Verification items for the finished model (mm, model axes). A direction names the side the tool comes from. Coordinates: 2 decimals unless noted, no trailing zeros. Write each loop counter-clockwise with the first axis right and the second up, starting at its lowest first coordinate (ties: lowest second). Pieces come first, ordered by that corner, then holes. Notation, with made-up numbers: (8.5, 22.25) -> (67.5, 22.25) arc R22 cw to (67.5, 39.25) -> close; hole circle Ø6 at (42, -28). An arc over 180 degrees is marked (long way). Write item = value, one per line. Start each with the question number.
(1) Mould release check, pull along Y, two halves, no side actions. Record for faces 4 (the face through (-40, -30, 12)), 5 (the face through (1, 9, 9.541)), 6 (the face through (-13, -49.9, 12.3)), 7 (the face through (-4, 43, 25)): released by +Y, released by -Y, zero draft, split by the parting line, or undercut.
(2) Set-up check for faces 1 (the face through (51.47, -0.38, 12.32)), 2 (the face through (-49.56, 6.61, 12.32)), 3 (the face through (44.387, -26.066, 12.325)): record each of +Z, -Z, +X, -X, +Y, -Y from which the full face is reachable in a straight line by a thin tool's end or side.
(3) Section check B-B (z = 18). State how many separate pieces and enclosed holes the cut face has, plus the area to 3 significant figures.
(4) Section check A-A (y = -30). Record the cut outline in (x, z), plus the area to 3 significant figures.
(5) Material ranges on probe 1 along X at (y, z) = (36, 24.5); probe 2 along Y at (x, z) = (3, 20.5); probe 3 along X at (y, z) = (44.5, 6), recorded low to high. Write a range as [from, to].
(6) Section check C-C (y = 5). Record the cut outline in (x, z).
(7) Gauge pin test, flat ends, axial feed: pin 1 Ø23 at (x, y) = (0, 25) entering from -Z; pin 2 Ø5 at (y, z) = (22.5, 22) entering from +X; pin 3 Ø10 at (x, z) = (-21, 7.5) entering from +Y. Record the tip position at first contact, or that the pin passes through.
```python
from build123d import *

# Parameters (mm, degrees)
SKETCH1_R           = 50
BOSS_EXTRUDE1_DEPTH = 25
SKETCH2_W           = 9.541105513
SKETCH2_H           = 36
SKETCH2_W_2         = 12.5
SKETCH2_4_W         = 9.541105513
SKETCH2_4_H         = 36
SKETCH2_4_W_2       = 12.5
SKETCH5_W           = 5
SKETCH5_H           = 7
SKETCH6_W           = 2
SKETCH6_H           = 9
SKETCH7_R           = 10
CUT_EXTRUDE1_DEPTH  = 74.610911988
BOSS_EXTRUDE2_DEPTH = 25
CIRPATTERN1_DEPTH   = 25


# Read off the part's stored shape, not the designer's step: CirPattern1
with BuildPart() as part:
    # Sketch1 → Boss-Extrude1 (new body)
    with BuildSketch(Plane.XY):
        Circle(SKETCH1_R)
    extrude(amount=BOSS_EXTRUDE1_DEPTH)

    # Sketch2 → Revolve1 (revolve)
    with BuildSketch(Plane(origin=(0, 0, 0), x_dir=(0, 0, -1), z_dir=(1, 0, 0))):
        with Locations((-4.770552756, -25)):
            Rectangle(SKETCH2_W, SKETCH2_H)
        with Locations((-18.75, -25)):
            Rectangle(SKETCH2_W_2, SKETCH2_H)
    revolve(axis=Axis((0, 0, -54.580519766), (0, 0, 1)))

    # Sketch2<4> → Cut-Revolve1 (revolve, cut)
    with BuildSketch(Plane(origin=(0, 0, 0), x_dir=(0, 0, -1), z_dir=(1, 0, 0)), mode=Mode.PRIVATE) as cut_revolve1_sk:
        with Locations((-4.770552756, -25)):
            Rectangle(SKETCH2_4_W, SKETCH2_4_H)
        with Locations((-18.75, -25)):
            Rectangle(SKETCH2_4_W_2, SKETCH2_4_H)
    revolve(cut_revolve1_sk.sketch.rotate(Axis((0, 0, -54.580519766), (0, 0, 1)), 270), axis=Axis((0, 0, -54.580519766), (0, 0, 1)), mode=Mode.SUBTRACT)

    # Sketch5 → Revolve3 (revolve)
    with BuildSketch(Plane(origin=(0, 0, 0), x_dir=(0, 0, -1), z_dir=(1, 0, 0)), mode=Mode.PRIVATE) as revolve3_sk:
        with Locations((-27.5, -3.5)):
            Rectangle(SKETCH5_W, SKETCH5_H)
    revolve(revolve3_sk.sketch.rotate(Axis((0, 0, 64.707463348), (0, 0, -1)), 90), axis=Axis((0, 0, 64.707463348), (0, 0, -1)))

    # Sketch6 → Cut-Revolve2 (revolve, cut)
    with BuildSketch(Plane(origin=(0, 0, 0), x_dir=(0, 0, -1), z_dir=(1, 0, 0)), mode=Mode.PRIVATE) as cut_revolve2_sk:
        with Locations((-1, -4.5)):
            Rectangle(SKETCH6_W, SKETCH6_H)
    revolve(cut_revolve2_sk.sketch.rotate(Axis((0, 0, -41.001610393), (0, 0, 1)), 270), axis=Axis((0, 0, -41.001610393), (0, 0, 1)), mode=Mode.SUBTRACT)

    # Sketch7 → Cut-Extrude1 (cut, through all)
    with BuildSketch(Plane(origin=(0, 0, 9.541105513), x_dir=(-1, 0, 0), z_dir=(0, 0, -1))):
        with Locations((0, 25)):
            Circle(SKETCH7_R)
        with Locations((21.650635095, 12.5)):
            Circle(SKETCH7_R)
        with Locations((21.650635095, -12.5)):
            Circle(SKETCH7_R)
        with Locations((0, -25)):
            Circle(SKETCH7_R)
        with Locations((-21.650635095, -12.5)):
            Circle(SKETCH7_R)
        with Locations((-21.650635095, 12.5)):
            Circle(SKETCH7_R)
    extrude(amount=-CUT_EXTRUDE1_DEPTH, mode=Mode.SUBTRACT)

    # Sketch8 → Boss-Extrude2 (add)
    with BuildSketch(Plane(origin=(0, 0, 0), x_dir=(-1, 0, 0), z_dir=(0, 0, -1))):
        with BuildLine():
            Line((-0.75, 49.994374684), (0, 52.994374684))
            Line((0, 52.994374684), (0.75, 49.994374684))
            ThreePointArc((0.75, 49.994374684), (0, 50), (-0.75, 49.994374684))
        make_face()
    extrude(amount=-BOSS_EXTRUDE2_DEPTH)

    # CirPattern1 outline → CirPattern1 (add)
    with BuildSketch(Plane.XY):
        with BuildLine():
            Line((-12.215051946, 48.48497196), (-13.715953451, 51.188635155))
            Line((-13.715953451, 51.188635155), (-13.663940686, 48.096743393))
            ThreePointArc((-13.663940686, 48.096743393), (-12.940952255, 48.296291315), (-12.215051946, 48.48497196))
        make_face()
        with BuildLine():
            ThreePointArc((12.215051946, 48.48497196), (12.940952255, 48.296291315), (13.663940686, 48.096743393))
            Line((13.663940686, 48.096743393), (13.715953451, 51.188635155))
            Line((13.715953451, 51.188635155), (12.215051946, 48.48497196))
        make_face()
        with BuildLine():
            ThreePointArc((24.347668289, 43.671398523), (25, 43.301270189), (25.646706395, 42.921398522))
            Line((25.646706395, 42.921398522), (26.497187342, 45.894474734))
            Line((26.497187342, 45.894474734), (24.347668289, 43.671398523))
        make_face()
        with BuildLine():
            ThreePointArc((34.821031274, 35.881691446), (35.35533906, 35.35533906), (35.881691446, 34.821031274))
            Line((35.881691446, 34.821031274), (37.472681703, 37.472681703))
            Line((37.472681703, 37.472681703), (34.821031274, 35.881691446))
        make_face()
        with BuildLine():
            ThreePointArc((42.921398522, 25.646706395), (43.301270189, 25), (43.671398522, 24.347668289))
            Line((43.671398522, 24.347668289), (45.894474734, 26.497187342))
            Line((45.894474734, 26.497187342), (42.921398522, 25.646706395))
        make_face()
        with BuildLine():
            ThreePointArc((48.096743392, 13.663940686), (48.296291315, 12.940952255), (48.48497196, 12.215051946))
            Line((48.48497196, 12.215051946), (51.188635155, 13.715953451))
            Line((51.188635155, 13.715953451), (48.096743392, 13.663940686))
        make_face()
        with BuildLine():
            ThreePointArc((49.994374684, 0.75), (50, 0), (49.994374684, -0.75))
            Line((49.994374684, -0.75), (52.994374684, 0))
            Line((52.994374684, 0), (49.994374684, 0.75))
        make_face()
        with BuildLine():
            ThreePointArc((48.48497196, -12.215051946), (48.296291315, -12.940952255), (48.096743392, -13.663940686))
            Line((48.096743392, -13.663940686), (51.188635155, -13.715953451))
            Line((51.188635155, -13.715953451), (48.48497196, -12.215051946))
        make_face()
        with BuildLine():
            ThreePointArc((43.671398522, -24.347668289), (43.301270189, -25), (42.921398522, -25.646706395))
            Line((42.921398522, -25.646706395), (45.894474734, -26.497187342))
            Line((45.894474734, -26.497187342), (43.671398522, -24.347668289))
        make_face()
        with BuildLine():
            ThreePointArc((35.881691446, -34.821031274), (35.355339059, -35.355339059), (34.821031274, -35.881691446))
            Line((34.821031274, -35.881691446), (37.472681703, -37.472681703))
            Line((37.472681703, -37.472681703), (35.881691446, -34.821031274))
        make_face()
        with BuildLine():
            ThreePointArc((25.646706395, -42.921398522), (25, -43.301270189), (24.347668289, -43.671398522))
            Line((24.347668289, -43.671398522), (26.497187342, -45.894474734))
            Line((26.497187342, -45.894474734), (25.646706395, -42.921398522))
        make_face()
        with BuildLine():
            ThreePointArc((13.663940686, -48.096743392), (12.940952255, -48.296291314), (12.215051946, -48.48497196))
            Line((12.215051946, -48.48497196), (13.715953451, -51.188635155))
            Line((13.715953451, -51.188635155), (13.663940686, -48.096743392))
        make_face()
        with BuildLine():
            ThreePointArc((0.75, -49.994374684), (0, -50), (-0.75, -49.994374684))
            Line((-0.75, -49.994374684), (0, -52.994374684))
            Line((0, -52.994374684), (0.75, -49.994374684))
        make_face()
        with BuildLine():
            ThreePointArc((-12.215051946, -48.48497196), (-12.940952255, -48.296291314), (-13.663940686, -48.096743392))
            Line((-13.663940686, -48.096743392), (-13.715953451, -51.188635155))
            Line((-13.715953451, -51.188635155), (-12.215051946, -48.48497196))
        make_face()
        with BuildLine():
            ThreePointArc((-24.347668289, -43.671398522), (-25, -43.301270189), (-25.646706395, -42.921398522))
            Line((-25.646706395, -42.921398522), (-26.497187342, -45.894474734))
            Line((-26.497187342, -45.894474734), (-24.347668289, -43.671398522))
        make_face()
        with BuildLine():
            ThreePointArc((-34.821031274, -35.881691446), (-35.355339059, -35.355339059), (-35.881691446, -34.821031274))
            Line((-35.881691446, -34.821031274), (-37.472681703, -37.472681703))
            Line((-37.472681703, -37.472681703), (-34.821031274, -35.881691446))
        make_face()
        with BuildLine():
            ThreePointArc((-42.921398522, -25.646706395), (-43.301270189, -25), (-43.671398522, -24.347668289))
            Line((-43.671398522, -24.347668289), (-45.894474734, -26.497187342))
            Line((-45.894474734, -26.497187342), (-42.921398522, -25.646706395))
        make_face()
        with BuildLine():
            ThreePointArc((-48.096743392, -13.663940686), (-48.296291315, -12.940952255), (-48.48497196, -12.215051946))
            Line((-48.48497196, -12.215051946), (-51.188635155, -13.715953451))
            Line((-51.188635155, -13.715953451), (-48.096743392, -13.663940686))
        make_face()
        with BuildLine():
            ThreePointArc((-49.994374684, -0.75), (-50, 0), (-49.994374684, 0.75))
            Line((-49.994374684, 0.75), (-52.994374684, 0))
            Line((-52.994374684, 0), (-49.994374684, -0.75))
        make_face()
        with BuildLine():
            ThreePointArc((-48.48497196, 12.215051946), (-48.296291315, 12.940952255), (-48.096743392, 13.663940686))
            Line((-48.096743392, 13.663940686), (-51.188635155, 13.715953451))
            Line((-51.188635155, 13.715953451), (-48.48497196, 12.215051946))
        make_face()
        with BuildLine():
            ThreePointArc((-43.671398522, 24.347668289), (-43.301270189, 25), (-42.921398522, 25.646706395))
            Line((-42.921398522, 25.646706395), (-45.894474734, 26.497187342))
            Line((-45.894474734, 26.497187342), (-43.671398522, 24.347668289))
        make_face()
        with BuildLine():
            ThreePointArc((-35.881691446, 34.821031274), (-35.35533906, 35.35533906), (-34.821031274, 35.881691446))
            Line((-34.821031274, 35.881691446), (-37.472681703, 37.472681703))
            Line((-37.472681703, 37.472681703), (-35.881691446, 34.821031274))
        make_face()
        with BuildLine():
            ThreePointArc((-25.646706395, 42.921398522), (-25, 43.301270189), (-24.347668289, 43.671398523))
            Line((-24.347668289, 43.671398523), (-26.497187342, 45.894474734))
            Line((-26.497187342, 45.894474734), (-25.646706395, 42.921398522))
        make_face()
    extrude(amount=CIRPATTERN1_DEPTH)


solid = part.part
```
Response:
q1.face_4 = undercut
q1.face_5 = undercut
q1.face_6 = released by -Y
q1.face_7 = zero draft
q2.face_1 = +Z, -Z, +X
q2.face_2 = +Z, -Z, -X
q2.face_3 = +Z, -Z, -Y
q3.separate_pieces = 2
q3.enclosed_holes = 1
q3.area = 2,250 mm2
q4.outline = (-40, 0) -> (-30.81, 0) -> (-30.81, 9.54) -> (-8.66, 9.54) -> (-8.66, 12.5) -> (-30.81, 12.5) -> (-30.81, 25) -> (-40, 25) -> close; (8.66, 9.54) -> (30.81, 9.54) -> (30.81, 0) -> (40, 0) -> (40, 25) -> (30.81, 25) -> (30.81, 12.5) -> (8.66, 12.5) -> close
q4.area = 591 mm2
q5.probe_1 = [-36.59, -35.02], [-34.7, -23.52], [23.52, 34.7], [35.02, 36.59]
q5.probe_2 = [-49.91, -42.9], [-6.32, 6.32], [42.9, 49.91]
q5.probe_3 = [-26.1, -25.15], [-22.8, 22.8], [25.15, 26.1]
q6.outline = (-49.75, 0) -> (-42.71, 0) -> (-42.71, 9.54) -> (-28.27, 9.54) -> (-28.27, 12.5) -> (-42.71, 12.5) -> (-42.71, 25) -> (-49.75, 25) -> close; (-15.04, 9.54) -> (-4.9, 9.54) -> (-4.9, 2) -> (4.9, 2) -> (4.9, 9.54) -> (15.04, 9.54) -> (15.04, 12.5) -> (4.9, 12.5) -> (4.9, 30) -> (-4.9, 30) -> (-4.9, 12.5) -> (-15.04, 12.5) -> close; (28.27, 9.54) -> (42.71, 9.54) -> (42.71, 0) -> (49.75, 0) -> (49.75, 25) -> (42.71, 25) -> (42.71, 12.5) -> (28.27, 12.5) -> close
q7.pin_1 = 9.54
q7.pin_2 = 45.83
q7.pin_3 = 47.37
